```python
from build123d import *

# Parameters (mm, degrees)
CYLINDER_R     = 1.5
CYLINDER_DEPTH = 5
BOX009_W       = 7
BOX009_H       = 7
BOX009_DEPTH   = 5


with BuildPart() as screwhole:
    # Cylinder → Cylinder (new body)
    with BuildSketch(Plane(origin=(3.5, 8.5, -5), x_dir=(1, 0, 0), z_dir=(0, 0, 1))):
        Circle(CYLINDER_R)
    extrude(amount=CYLINDER_DEPTH)


with BuildPart() as cut005:
    # Box009 → Box009 (new body)
    with BuildSketch(Plane(origin=(0, 5, -5), x_dir=(1, 0, 0), z_dir=(0, 0, 1))):
        with Locations((3.5, 3.5)):
            Rectangle(BOX009_W, BOX009_H)
    extrude(amount=BOX009_DEPTH)

    # Cut005: cut ScrewHole
    add(screwhole.part, mode=Mode.SUBTRACT)


solid = cut005.part
```
Can you work these out from the model? Positions are in its coordinate system, mm. Give positions to 0.01 mm unless a question says otherwise; leave off trailing zeros. Loops run counter-clockwise (first coordinate to the right, second up) from the corner with the lowest first, then second, coordinate; pieces in that order, holes last. Notation, with made-up numbers: M 2,33.25 L 48,33.25 A25 cw 48,63.25 Z; hole C 3.5,37 d1. An arc over 180 degrees is marked long. Use one line per item in the form item = value. Start each with the question number.
(1) I want a section at A-A, the plane x = 3.5. Write out the boundary of the cut face in (y, z).
(2) I want a section at B-B, the plane y = 8.5. Write out the boundary of the cut face in (x, z), and give its area (3 significant figures).
(3) Please list where these lines run through material, in increasing order: line 1 (Y direction, x = 3.5, z = -3.1); line 2 (Y direction, x = 3, z = -4.5); line 3 (X direction, y = 8.25, z = -0.4).
(4) I want a section at C-C, the plane z = -2.05. Write out the boundary of the cut face in (x, y), and give its area (3 significant figures).
(5) Thinking about a two-plate mould opening in X: for faces 1 (the flat face through (2.7, 7, 0)), 2 (the flat face through (0, 8, -3)), 3 (the cylindrical face through (4.19, 7.17, -2.54)), which applies, released by +X, released by -X, zero draft, split by the parting line, or undercut?
Worked out:
q1.outline = M 5,-5 L 7,-5 L 7,0 L 5,0 Z; M 10,-5 L 12,-5 L 12,0 L 10,0 Z
q2.outline = M 0,-5 L 2,-5 L 2,0 L 0,0 Z; M 5,-5 L 7,-5 L 7,0 L 5,0 Z
q2.area = 20.0 mm²
q3.line_1 = 5 to 7, 10 to 12
q3.line_2 = 5 to 7.09, 9.91 to 12
q3.line_3 = 0 to 2.02, 4.98 to 7
q4.outline = M 0,5 L 7,5 L 7,12 L 0,12 Z; hole C 3.5,8.5 d3
q4.area = 41.9 mm²
q5.face_1 = zero draft
q5.face_2 = released by -X
q5.face_3 = undercut
